Autodesk Inventor part; units mm, degrees
ref_plane "Plano de trabajo1" through (30, 55, 0) normal (0, 0, -1) x (-1, 0, 0)
ref_plane "YZ Plane" through (0, 0, 0) normal (1, 0, 0) x (0, 1, 0)
ref_plane "XZ Plane" through (0, 0, 0) normal (0, 1, 0) x (-1, 0, 0)
sketch "Boceto2" plane through (0, 0, 0) normal (0, 1, 0) x (-1, 0, 0)
  line L0 (-30, 100) -> (30, 100)
  line L1 (30, 100) -> (30, -100)
  line L2 (30, -100) -> (-30, -100)
  line L3 (-30, -100) -> (-30, 100)
  line L4 (-30, 100) -> (30, -100) construction
  line L5 (30, 100) -> (-30, -100) construction
  point P0 (0, 0)
  dimension "d0" = 60
  dimension "d1" = 200
extrude "Extrusión1" add sketch "Boceto2" along normal blind 55
sketch "Boceto3" plane through (30, 0, -100) normal (0, 0, -1) x (-1, 0, 0)
  line L0 (7.5, 50) -> (52.5, 50)
  line L1 (52.5, 50) -> (52.5, 0)
  line L2 (52.5, 0) -> (7.5, 0)
  line L3 (7.5, 0) -> (7.5, 50)
  line L4 (0, 0) -> (60, 0)
  point P0 (30, 0)
  dimension "d4" = 45
  dimension "d5" = 50
  dimension "d6" = 0
extrude "Extrusión2" cut sketch "Boceto3" against normal blind 190
sketch "Boceto4" plane through (30, 0, 100) normal (1, 0, 0) x (0, 0, -1)
  line L0 (10, 50) -> (10, 0)
  line L1 (10, 50) -> (10, 0)
  line L2 (200, 0) -> (0, 0)
  line L3 (10, 50) -> (10, 0)
  line L4 (190, 0) -> (190, 50)
  line L5 (200, 50) -> (10, 50)
  line L6 (200, 0) -> (200, 55)
  line L7 (10, 15) -> (190, 15)
  line L8 (10, 50) -> (190, 50)
  point P0 (100, 0)
  point P1 (200, 27.5)
  dimension "d9" = 10
  dimension "d10" = 15
extrude "Extrusión3" cut sketch "Boceto4" against normal blind 10 contours L5 L4 L7 L0
sketch "Boceto5" plane through (0, 0, 0) normal (0, 1, 0) x (-1, 0, 0)
  line L0 (30, -100) -> (30, 100)
  line L1 (30, 0) -> (60, 0)
  line L2 (90, 30) -> (30, 30)
  line L3 (30, 30) -> (30, -30)
  line L4 (30, -30) -> (90, -30)
  line L5 (90, -30) -> (90, 30)
  line L6 (90, 30) -> (30, -30) construction
  line L7 (30, 30) -> (90, -30) construction
  circle A0 centre (50, 11.5) radius 3.25
  circle A1 centre (50, -11.5) radius 3.25
  circle A2 centre (80, 11.5) radius 3.25
  circle A3 centre (80, -11.5) radius 3.25
  point P0 (0, 0)
  dimension "d16" = 30
  dimension "d17" = 60
  dimension "d18" = 60
  dimension "d19" = 6.5
  dimension "d20" = 20
  dimension "d21" = 18.5
  dimension "d22" = 23
  dimension "d23" = 6.5
  dimension "d24" = 30
  dimension "d25" = 18.5
extrude "Extrusión4" add sketch "Boceto5" along normal blind 10
sketch "Boceto6" plane through (0, 55, 0) normal (0, 1, 0) x (1, 0, 0)
  line L0 (-30, 30) -> (-30, -30)
  line L1 (30, -14) -> (-30, -14)
  line L2 (-30, -14) -> (-30, 14)
  line L3 (-30, 14) -> (30, 14)
  line L4 (30, 14) -> (30, -14)
  line L5 (30, -14) -> (-30, 14) construction
  line L6 (-30, -14) -> (30, 14) construction
  point P0 (0, 0)
  dimension "d28" = 28
extrude "Extrusión5" add sketch "Boceto6" along normal blind 40
sketch "Boceto7" plane through (0, 95, 0) normal (0, 1, 0) x (1, 0, 0)
  line L0 (-23.5, 11) -> (23.5, 11)
  line L1 (23.5, 11) -> (23.5, -11)
  line L2 (23.5, -11) -> (-23.5, -11)
  line L3 (-23.5, -11) -> (-23.5, 11)
  line L4 (-23.5, 11) -> (23.5, -11) construction
  line L5 (23.5, 11) -> (-23.5, -11) construction
  point P0 (0, 0)
  dimension "d31" = 47
  dimension "d32" = 22
extrude "Extrusión6" cut sketch "Boceto7" against normal blind 43
sketch "Boceto8" plane through (-30, 0, 100) normal (-1, 0, 0) x (0, 0, 1)
  line L0 (-200, 55) -> (-114, 55)
  line L1 (0, 55) -> (-86, 55)
  line L2 (-114, 55) -> (-86, 55)
  line L3 (-111, 65) -> (-89, 65)
  line L4 (-89, 65) -> (-89, 55)
  line L5 (-89, 55) -> (-111, 55)
  line L6 (-111, 55) -> (-111, 65)
  line L7 (-111, 65) -> (-89, 55) construction
  line L8 (-89, 65) -> (-111, 55) construction
  point P0 (-100, 0)
  point P1 (-100, 60)
  dimension "d35" = 22
  dimension "d36" = 10
  dimension "d37" = 0
extrude "Extrusión7" cut sketch "Boceto8" against normal blind 10
ref_plane "Plano de trabajo1" through (30, 55, 0) normal (0, 0, -1) x (-1, 0, 0)
sketch "Boceto10" plane through (30, 55, 0) normal (0, 0, -1) x (-1, 0, 0)
  line L0 (60.12, -45) -> (60.12, 17.4198)
  line L1 (60.12, -45) -> (60.12, 13.5667)
  line L2 (60.12, -45) -> (137.1989, -45)
  line L3 (60.12, -19.9519) -> (80.5233, -61.6073)
  line L4 (120, -45) -> (60, -45)
  point P0 (30, -55)
  point P1 (72.3889, -45)
  dimension "d41" = 0
extrude "Extrusión8" add sketch "Boceto10" along normal mid plane 15
properties part number "depth_camera_support"
The model under review builds one solid part; all positions refer to its coordinate system, in mm. A direction names the side the tool comes from. Round coordinates to 2 decimals unless told otherwise and drop trailing zeros. Order: outer loops, then holes, each group sorted by start corner. A loop starts at its lowest first (then second) coordinate and runs counter-clockwise, first axis right, second up.
Item 1: Add section C-C, the plane x = -80. State the section outline as (y, z) points.
Working result:
outline: (0, -30) - (10, -30) - (10, -14.75) - (0, -14.75) - close; (0, -8.25) - (10, -8.25) - (10, 8.25) - (0, 8.25) - close; (0, 14.75) - (10, 14.75) - (10, 30) - (0, 30) - close
Item 2: Machinability: for faces 1 (the flat face through (30, 12, 7)), 2 (the cylindrical face through (-76.753, 4.93, 11.357)), 3 (the flat face through (-27, 55, 0)), 4 (the flat face through (-60, 5, 30)), 5 (the flat face through (26, 32, -90)), which of the approach directions +Z, -Z, +X, -X, +Y, -Y give a long, thin tool a straight path to every point of the face, cutting with its end or side? Answer none if there is none.
Working result:
face 1: +Z, -Z, +X, +Y, -Y
face 2: +Y, -Y
face 3: -X
face 4: +Z, -X, +Y, -Y
face 5: +X
Item 3: To check wall thickness, follow probe 1 along Z at (x, y) = (-80, 4.75); probe 2 along Y at (x, z) = (-59, 1); probe 3 along Z at (x, y) = (-5, 87). State the ranges of each line that lie inside material, in increasing order.
Working result:
probe 1: z = -30 to -14.75, -8.25 to 8.25, 14.75 to 30
probe 2: y = 0 to 10
probe 3: z = -14 to -11, 11 to 14
Item 4: Add section A-A, the plane z = 18.5. State the section outline as (x, y) points, and give its area (3 significant figures).
Working result:
outline: (-90, 0) - (-22.5, 0) - (-22.5, 50) - (30, 50) - (30, 55) - (-30, 55) - (-30, 10) - (-90, 10) - close; (22.5, 0) - (30, 0) - (30, 15) - (22.5, 15) - close
area: 1,390 mm2
Item 5: Draft analysis for pull direction Z (two halves, no side actions). For faces 6 (the flat face through (0, 95, 12)), 7 (the flat face through (-60, 5, -30)), 8 (the flat face through (23.5, 74, 0)), 9 (the flat face through (0, 52, 0)), state which applies: released by +Z, released by -Z, zero draft, split by the parting line, or undercut.
Working result:
face 6: zero draft
face 7: released by -Z
face 8: undercut
face 9: undercut
Item 6: Add section B-B, the plane y = 87.5. State the section outline as (x, z) points.
Working result:
outline: (-30, -14) - (30, -14) - (30, 14) - (-30, 14) - close; hole (-23.5, -11) - (23.5, -11) - (23.5, 11) - (-23.5, 11) - close
Item 7: For pin 1 (12 mm diameter, centred on x = -0.5, y = 27.5, fed in from -Z); pin 2 (4.5 mm diameter, centred on y = 24.5, z = 0.5, fed in from +X); pin 3 (20 mm diameter, centred on x = -5.5, y = 80, fed in from +Z), all flat-tipped, find the tip position at first contact; note any pin that passes through.
Working result:
pin 1: stops at z = 90
pin 2: stops at x = -22.5
pin 3: stops at z = 14
Item 8: Add section D-D, the plane y = 21. State the section outline as (x, z) points, and give its area (3 significant figures).
Working result:
outline: (-37, -7.5) - (-30.12, -7.5) - (-30.12, 7.5) - (-37, 7.5) - close; (-30, -100) - (-22.5, -100) - (-22.5, 90) - (30, 90) - (30, 100) - (-30, 100) - close; (22.5, -100) - (30, -100) - (30, -90) - (22.5, -90) - close
area: 2,200 mm2
